from build123d import *

# Parameters (mm, degrees)
BOSS_EXTRUDE1_DEPTH = 5.08
SKETCH2_W           = 6.9215
SKETCH2_H           = 203.2
BOSS_EXTRUDE2_DEPTH = 2.54


with BuildPart() as part:
    # Sketch1 → Boss-Extrude1 (new body)
    with BuildSketch(Plane(origin=(0, 0, 0), x_dir=(0, 0, -1), z_dir=(1, 0, 0))):
        Polygon((-3.048, 15.875), (-7.9375, 15.875), (-7.9375, 219.075), (-3.048, 219.075), (-3.048, 222.885), (-5.588, 222.885), (-5.588, 227.965), (0, 224.155), (5.588, 227.965), (5.588, 222.885), (3.048, 222.885), (3.048, 219.075), (7.9375, 219.075), (7.9375, 15.875), (3.048, 15.875), (3.048, 12.065), (5.588, 12.065), (5.588, 6.985), (0, 10.795), (-5.588, 6.985), (-5.588, 12.065), (-3.048, 12.065), align=None)
    extrude(amount=BOSS_EXTRUDE1_DEPTH)

    # Sketch2 → Boss-Extrude2 (add)
    with BuildSketch(Plane(origin=(5.08, 0, 0), x_dir=(0, 0, -1), z_dir=(1, 0, 0))):
        with Locations((4.47675, 117.475)):
            Rectangle(SKETCH2_W, SKETCH2_H)
        with Locations((-4.47675, 117.475)):
            Rectangle(SKETCH2_W, SKETCH2_H)
    extrude(amount=BOSS_EXTRUDE2_DEPTH)


solid = part.part
Build history of the part. All positions in model axes, mm. A direction names the side the tool comes from. Coordinates: 2 decimals unless noted, no trailing zeros. Write each loop counter-clockwise with the first axis right and the second up, starting at its lowest first coordinate (ties: lowest second). Pieces come first, ordered by that corner, then holes. Notation, with made-up numbers: (-6.75, 85.25) -> (35.25, 85.25) arc R28 ccw to (35.25, 120.25) -> close; hole circle Ø2 at (72.25, 7). An arc over 180 degrees is marked (long way). Use CSV: the item, a comma, the result in double quotes. Start each with the question number.
Q1. Drill centre lines: probe 1 along Z at (x, y) = (7, 43); probe 2 along Y at (x, z) = (3, -5.25) (3 decimals); probe 3 along Y at (x, z) = (4.5, 4.25) (3 decimals). Where is each one in solid material? Low to high.
Q2. Cut at B-B, the plane y = 24. List the corners of the cut face in (x, z), then the cut area to 3 significant figures.
Q3. Cut at A-A, the plane x = 3.5. List the corners of the cut face in (y, z) (1 decimal), then the cut area to 3 significant figures.
Q4. Pull direction Y, two halves, no side cores. Call faces 1 (the flat face through (4, 15.875, 5)), 2 (the flat face through (3, 225, 5.588)), 3 (the flat face through (2.504, 8.863, -2.833)): released by +Y, released by -Y, zero draft, split by the parting line, or undercut.
Q5. Flat gauge pins, fed straight in: pin 1 Ø2 at (x, z) = (2.5, 4.5) entering from +Y (3 decimals); pin 2 Ø2 at (x, z) = (3, 0.5) entering from -Y; pin 3 Ø1.1 at (x, y) = (2, 14) entering from -Z. Where does each tip first touch, or does it go through?
Q6. 3-axis set-ups, long thin cutter, end or side, ignore diameter. For faces 4 (the flat face through (2.5, 226.03, -2.75)), 5 (the flat face through (3, 10, -5.588)), 6 (the flat face through (4, 219.075, 5)), 7 (the flat face through (3, 225, -5.588)): which of +Z, -Z, +X, -X, +Y, -Y reach the whole face in a straight line?
Checked values:
1,probe 1,"z = -7.94 to -1.02, 1.02 to 7.94"
1,probe 2,"y = 7.215 to 12.065, 15.875 to 219.075, 222.885 to 227.735"
1,probe 3,"y = 7.897 to 12.065, 15.875 to 219.075, 222.885 to 227.053"
2,outline,"(0, -7.94) -> (7.62, -7.94) -> (7.62, -1.02) -> (5.08, -1.02) -> (5.08, 1.02) -> (7.62, 1.02) -> (7.62, 7.94) -> (0, 7.94) -> close"
2,area,"116 mm²"
3,outline,"(7, -5.6) -> (12.1, -5.6) -> (12.1, -3) -> (15.9, -3) -> (15.9, -7.9) -> (219.1, -7.9) -> (219.1, -3) -> (222.9, -3) -> (222.9, -5.6) -> (228, -5.6) -> (224.2, 0) -> (228, 5.6) -> (222.9, 5.6) -> (222.9, 3) -> (219.1, 3) -> (219.1, 7.9) -> (15.9, 7.9) -> (15.9, 3) -> (12.1, 3) -> (12.1, 5.6) -> (7, 5.6) -> (10.8, 0) -> close"
3,area,"3,340 mm²"
4,face 1,"undercut"
4,face 2,"zero draft"
4,face 3,"released by -Y"
5,pin 1,"stops at y = 227.905"
5,pin 2,"stops at y = 9.77"
5,pin 3,"stops at z = -3.05"
6,face 4,"+X, -X, +Y"
6,face 5,"-Z, +X, -X, -Y"
6,face 6,"+Z, +X"
6,face 7,"-Z, +X, -X, +Y"
